from build123d import *

# Parameters (mm, degrees)
BOSS_EXTRUDE1_DEPTH     = 9.6139
SKETCH2_R               = 4.99745
CUT_EXTRUDE1_DEPTH      = 1
CUT_EXTRUDE1_DEPTH_BACK = 31.607
CUT_EXTRUDE2_DEPTH      = 1
CUT_EXTRUDE2_DEPTH_BACK = 31.607


with BuildPart() as part:
    # Sketch1 → Boss-Extrude1 (new body, symmetric)
    with BuildSketch(Plane.XY):
        with BuildLine():
            Line((0, 0), (0, 88.4682))
            ThreePointArc((0, 88.4682), (15.3035, 103.7717), (30.607, 88.4682))
            Line((30.607, 88.4682), (30.607, 0))
            Line((30.607, 0), (27.6225, 0))
            Line((27.6225, 0), (27.6225, 88.4682))
            ThreePointArc((27.6225, 88.4682), (15.3035, 100.7872), (2.9845, 88.4682))
            Line((2.9845, 88.4682), (2.9845, 0))
            Line((2.9845, 0), (0, 0))
        make_face()
    extrude(amount=BOSS_EXTRUDE1_DEPTH, both=True)

    # Sketch2 → Cut-Extrude1 (cut, two sides)
    with BuildSketch(Plane(origin=(30.607, 0, 0), x_dir=(0, 0, -1), z_dir=(1, 0, 0))) as cut_extrude1_sk:
        with Locations((0, 11.63955)):
            Circle(SKETCH2_R)
    extrude(amount=CUT_EXTRUDE1_DEPTH, mode=Mode.SUBTRACT)
    extrude(cut_extrude1_sk.sketch, amount=-CUT_EXTRUDE1_DEPTH_BACK, mode=Mode.SUBTRACT)

    # Sketch2<3> → Cut-Extrude2 (cut, two sides)
    with BuildSketch(Plane(origin=(30.607, 0, 0), x_dir=(0, 0, -1), z_dir=(1, 0, 0))) as cut_extrude2_sk:
        with BuildLine():
            ThreePointArc((0, 0), (-5.182448154, 1.004775894), (-9.6139, 3.8735))
            Line((-9.6139, 3.8735), (-9.6139, 0))
            Line((-9.6139, 0), (0, 0))
        make_face()
        with BuildLine():
            ThreePointArc((9.6139, 3.8735), (5.182448154, 1.004775894), (0, 0))
            Line((0, 0), (9.6139, 0))
            Line((9.6139, 0), (9.6139, 3.8735))
        make_face()
    extrude(amount=CUT_EXTRUDE2_DEPTH, mode=Mode.SUBTRACT)
    extrude(cut_extrude2_sk.sketch, amount=-CUT_EXTRUDE2_DEPTH_BACK, mode=Mode.SUBTRACT)


solid = part.part
Could you check a few things on this model? Use its own coordinates, in mm. A direction names the side the tool comes from. Give positions to 0.01 mm unless a question says otherwise; leave off trailing zeros. Order: outer loops, then holes, each group sorted by start corner. A loop starts at its lowest first (then second) coordinate and runs counter-clockwise, first axis right, second up.
1. For pin 1 (6 mm diameter, centred on x = 25, y = 37.5, fed in from -Z); pin 2 (1.5 mm diameter, centred on x = 8, z = 6.5, fed in from +Y); pin 3 (1 mm diameter, centred on x = 24.5, z = -7, fed in from -Y); pin 4 (5 mm diameter, centred on x = 15, z = -4, fed in from -Y), each with a flat end and sliding along its axis, tell me the tip position at first contact or that it passes through.
Answers below:
pin 1: stops at z = -9.61
pin 2: stops at y = 102.3
pin 3: stops at y = 96.07
pin 4: stops at y = 100.46
2. Suppose I cut it at A-A (y = 32.5). Write out the boundary of the cut face in (x, z), plus the area to 3 significant figures.
Answers below:
outline: (0, -9.61) - (2.98, -9.61) - (2.98, 9.61) - (0, 9.61) - close; (27.62, -9.61) - (30.61, -9.61) - (30.61, 9.61) - (27.62, 9.61) - close
area: 115 mm2
3. Suppose I cut it at C-C (z = 7). Write out the boundary of the cut face in (x, y), plus the area to 3 significant figures.
Answers below:
outline: (0, 1.9) - (2.98, 1.9) - (2.98, 88.47) arc R12.32 cw to (27.62, 88.47) - (27.62, 1.9) - (30.61, 1.9) - (30.61, 88.47) arc R15.3 ccw to (0, 88.47) - close
area: 646 mm2
4. Suppose I cut it at B-B (z = 2.75). Write out the boundary of the cut face in (x, y), plus the area to 3 significant figures.
Answers below:
outline: (0, 0.28) - (2.98, 0.28) - (2.98, 7.47) - (0, 7.47) - close; (0, 15.81) - (2.98, 15.81) - (2.98, 88.47) arc R12.32 cw to (27.62, 88.47) - (27.62, 15.81) - (30.61, 15.81) - (30.61, 88.47) arc R15.3 ccw to (0, 88.47) - close; (27.62, 0.28) - (30.61, 0.28) - (30.61, 7.47) - (27.62, 7.47) - close
area: 606 mm2
5. Which directions (+Z, -Z, +X, -X, +Y, -Y) give clear straight access to the entire face, cutting with the end or side of a thin tool? Please do faces 1 (the cylindrical face through (14.97, 103.77, 0.13)), 2 (the flat face through (2.984, 45, 0)).
Answers below:
face 1: +Z, -Z, +Y
face 2: +Z, -Z, -Y
6. I need wall thicknesses on L1, parallel to X at y = 12, z = 8; L2, parallel to Y at x = 25, z = -0.75; L3, parallel to Y at x = 10.5, z = 3.75. Which ranges of each line are inside material? Lowest first, please.
Answers below:
L1: x = 0 to 2.98, 27.62 to 30.61
L2: y = 96.07 to 100.31
L3: y = 99.81 to 103
7. Suppose I cut it at D-D (y = 92.5). Write out the boundary of the cut face in (x, z).
Answers below:
outline: (0.54, -9.61) - (3.66, -9.61) - (3.66, 9.61) - (0.54, 9.61) - close; (26.94, -9.61) - (30.07, -9.61) - (30.07, 9.61) - (26.94, 9.61) - close
8. Thinking about a two-plate mould opening in Z: for faces 3 (the cylindrical face through (29.14, 6.76, 1.08)), 4 (the flat face through (28, 54, 9.614)), 5 (the flat face through (28, 54, -9.614)), 6 (the flat face through (30.607, 45, 0)), which applies, +Z half, -Z half, draft (parallel to the pull), parting line (faces both ways), or undercut?
Answers below:
face 3: undercut
face 4: +Z half
face 5: -Z half
face 6: draft
